Geometry: final body of the model. Coordinates: model frame, mm. Face numbers are marked on the shaded views. A direction names the side the tool comes from. Give positions to 0.01 mm unless a question says otherwise; leave off trailing zeros. Write each loop counter-clockwise with the first axis right and the second up, starting at its lowest first coordinate (ties: lowest second). Pieces come first, ordered by that corner, then holes. Notation, with made-up numbers: (30, 82) -> (58, 82) arc R23 ccw to (58, 106) -> close; hole circle Ø6 at (4.25, 59.25). An arc over 180 degrees is marked (long way). Answer in a Markdown table with one row per item. Add a question column.
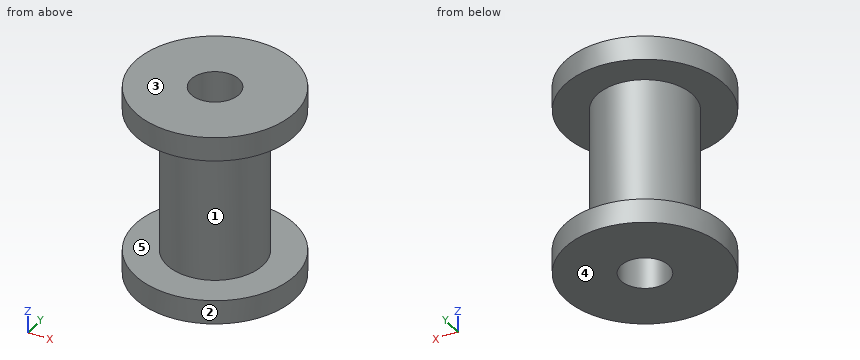
from build123d import *

# Parameters (mm, degrees)
EXTRUDE_1_DEPTH      = 4.5
EXTRUDE_1_DEPTH_BACK = 4.5
SKETCH_1_R           = 3
SKETCH_2_R           = 5
EXTRUDE_2_DEPTH      = 1.5
EXTRUDE_START        = 1.5
SKETCH_3_R           = 5
EXTRUDE_3_DEPTH      = 1.5
SKETCH_4_R           = 1.5
CUT_EXTRUDE_1_DEPTH  = 14.928388277


with BuildPart() as part:
    # Sketch 1 → Extrude 1 (new, two sides: drawn at the far end of the back side and taken through both)
    with BuildSketch(Plane.XY.offset(-EXTRUDE_1_DEPTH_BACK)):
        Circle(SKETCH_1_R)
    extrude(amount=EXTRUDE_1_DEPTH + EXTRUDE_1_DEPTH_BACK)

    # Sketch 2 → Extrude 2 (add)
    with BuildSketch(Plane.XY.offset(4.5)):
        Circle(SKETCH_2_R)
    extrude(amount=EXTRUDE_2_DEPTH)

    # Sketch 3 → Extrude 3 (add)
    with BuildSketch(Plane(origin=(0, 0, -4.5), x_dir=(-1, 0, 0), z_dir=(0, 0, -1)).offset(EXTRUDE_START)):
        with Locations(Location((0, 0, 0), (0, 0, 180))):
            Circle(SKETCH_3_R)
    extrude(amount=-EXTRUDE_3_DEPTH)

    # Sketch 4 → Cut-Extrude 1 (cut, through all)
    with BuildSketch(Plane(origin=(0, 0, -6), x_dir=(-1, 0, 0), z_dir=(0, 0, -1))):
        Circle(SKETCH_4_R)
    extrude(amount=-CUT_EXTRUDE_1_DEPTH, mode=Mode.SUBTRACT)


solid = part.part
Q1. Pull-direction query (Z, two-part tool) for the marked faces 1, 2 and 3; classes: +Z half, -Z half, draft (parallel to the pull), parting line (faces both ways), or undercut.
Q2. Access query for the marked faces 4 and 5. Directions: +Z, -Z, +X, -X, +Y, -Y. A direction counts if a zero-diameter tool reaches every point of the face in a straight line with its end or side. Return the directions, or none.
Q3. Contact query for flat-ended pins moving along their axis: pin 1 Ø4 at (x, y) = (0, 0) entering from -Z; pin 2 Ø4 at (x, z) = (3.5, 4.5) entering from -Y; pin 3 Ø1 at (y, z) = (2.5, -3) entering from +X. Output: stop coordinate, or through.
Q4. Line query: probe 1 along Z at (x, y) = (-3.5, -1.5); probe 2 along Y at (x, z) = (0, -1.5); probe 3 along Y at (x, z) = (0.25, 5.5). Output: solid intervals per line, ascending. Write a range as from..to.
Q5. Section A-A on y = 0. Return loops of the section in (x, z).
Q6. Section D-D on x = 2.25. Return loops of the section in (y, z), and give its area (3 significant figures).
Q7. Section B-B on x = 0.5. Return loops of the section in (y, z), and give its area (3 significant figures).
Q8. Section C-C on z = -1.75. Return loops of the section in (x, y).
Checks:
| question | item | result |
|---|---|---|
| 1 | face 1 | undercut |
| 1 | face 2 | draft |
| 1 | face 3 | +Z half |
| 2 | face 4 | -Z, +X, -X, +Y, -Y |
| 2 | face 5 | none |
| 3 | pin 1 | z = -6 |
| 3 | pin 2 | y = -4.77 |
| 3 | pin 3 | x = 2.24 |
| 4 | probe 1 | -6..-4.5, 4.5..6 |
| 4 | probe 2 | -3..-1.5, 1.5..3 |
| 4 | probe 3 | -4.99..-1.48, 1.48..4.99 |
| 5 | outline | (-5, -6) -> (-1.5, -6) -> (-1.5, 6) -> (-5, 6) -> (-5, 4.5) -> (-3, 4.5) -> (-3, -4.5) -> (-5, -4.5) -> close; (1.5, -6) -> (5, -6) -> (5, -4.5) -> (3, -4.5) -> (3, 4.5) -> (5, 4.5) -> (5, 6) -> (1.5, 6) -> close |
| 6 | outline | (-4.47, -6) -> (4.47, -6) -> (4.47, -4.5) -> (1.98, -4.5) -> (1.98, 4.5) -> (4.47, 4.5) -> (4.47, 6) -> (-4.47, 6) -> (-4.47, 4.5) -> (-1.98, 4.5) -> (-1.98, -4.5) -> (-4.47, -4.5) -> close |
| 6 | area | 62.5 mm^2 |
| 7 | outline | (-4.97, -6) -> (-1.41, -6) -> (-1.41, 6) -> (-4.97, 6) -> (-4.97, 4.5) -> (-2.96, 4.5) -> (-2.96, -4.5) -> (-4.97, -4.5) -> close; (1.41, -6) -> (4.97, -6) -> (4.97, -4.5) -> (2.96, -4.5) -> (2.96, 4.5) -> (4.97, 4.5) -> (4.97, 6) -> (1.41, 6) -> close |
| 7 | area | 49.2 mm^2 |
| 8 | outline | circle Ø6 at (0, 0); hole circle Ø3 at (0, 0) |
